Read the model definition and answer for the solid it produces. Units are mm, in the model's axes. Face numbers are marked on the shaded views. Coordinates: 2 decimals unless noted, no trailing zeros. Write each loop counter-clockwise with the first axis right and the second up, starting at its lowest first coordinate (ties: lowest second). Pieces come first, ordered by that corner, then holes.
1) Determine the mould class of the marked faces 1, 2 and 3 for opening direction Z: +Z half, -Z half, draft (parallel to the pull), parting line (faces both ways), or undercut.
2) The part is cut by section B-B (x = -10). Determine the outline of the cut face in (y, z), then the cut area to 3 significant figures.
3) Find the intervals of material crossed by line 1 (X direction, y = 6.25, z = 13.5); line 2 (X direction, y = 6, z = 13.5); line 3 (Z direction, x = -6, y = 4.75), in increasing order.
4) Each of these flat-tipped pins is pushed along its axis until it touches: pin 1 Ø2 at (x, y) = (11.5, 7) entering from +Z; pin 2 Ø1.8 at (y, z) = (5.5, 10) entering from +X; pin 3 Ø1 at (y, z) = (6, 11) entering from -X. Where does it stop, or does it pass through?
5) The part is cut by section A-A (z = 10). Determine the outline of the cut face in (x, y), then the cut area to 3 significant figures.
from build123d import *

# Parameters (mm, degrees)
F0_W      = 40
F0_H      = 20
F1_DEPTH  = 20
F2_R      = 1.75
F3_DEPTH  = 15
F4_R      = 1.75
F5_DEPTH  = 15
F6_R      = 0.5
F7_DEPTH  = 20.001
F8_R      = 2
F9_DEPTH  = 2
F12_R     = 2
F13_DEPTH = 2


with BuildPart() as f1:
    # F0 (on Top) → F1 (new body)
    with BuildSketch(Plane.XY):
        with Locations((-0.4968201369, 6.2780210599)):
            Rectangle(F0_W, F0_H)
    extrude(amount=F1_DEPTH)

    # F2 (on face) → F3 (cut)
    with BuildSketch(Plane(origin=(-20.4968201369, 0, 0), x_dir=(0, -1, 0), z_dir=(-1, 0, 0))):
        with Locations((-6.2780210599, 10)):
            Circle(F2_R)
    extrude(amount=-F3_DEPTH, mode=Mode.SUBTRACT)

    # F4 (on face) → F5 (cut)
    with BuildSketch(Plane.YZ.offset(19.5031798631)):
        with Locations((6.2780210599, 10)):
            Circle(F4_R)
    extrude(amount=-F5_DEPTH, mode=Mode.SUBTRACT)

    # F6 (on face) → F7 (cut, through all)
    with BuildSketch(Plane.XY.offset(20)):
        with Locations((-12.9968201369, 6.2780210599)):
            Circle(F6_R)
        with Locations((12.9968201369, 6.2780210599)):
            Circle(F6_R)
    extrude(amount=-F7_DEPTH, mode=Mode.SUBTRACT)

    # F8 (on face) → F9 (cut)
    with BuildSketch(Plane.XY.offset(20)):
        with Locations((-12.9968201369, 6.2780210599)):
            Circle(F8_R)
    extrude(amount=-F9_DEPTH, mode=Mode.SUBTRACT)

    # F10 (on face) → F11 (revolve, cut)
    with BuildSketch(Plane.XY.offset(18)):
        with BuildLine():
            Line((-12.9968201369, 4.2780210599), (-12.9968201369, 8.2780210599))
            ThreePointArc((-12.9968201369, 8.2780210599), (-14.9968201369, 6.2780210599), (-12.9968201369, 4.2780210599))
        make_face()
    revolve(axis=Axis((-12.9968201369, 6.2780210599, 18), (0, -1, 0)), mode=Mode.SUBTRACT)

    # F12 (on face) → F13 (cut)
    with BuildSketch(Plane.XY.offset(20)):
        with Locations((12.9968201369, 6.2780210599)):
            Circle(F12_R)
    extrude(amount=-F13_DEPTH, mode=Mode.SUBTRACT)

    # F14 (on face) → F15 (revolve, cut)
    with BuildSketch(Plane.XY.offset(18)):
        with BuildLine():
            Line((13.0087840564, 4.278056844), (13.0087840564, 8.2779852757))
            ThreePointArc((13.0087840564, 8.2779852757), (11.0088198406, 6.2780210599), (13.0087840564, 4.278056844))
        make_face()
    revolve(axis=Axis((13.0087840564, 6.2780210599, 18), (0, -1, 0)), mode=Mode.SUBTRACT)


solid = f1.part
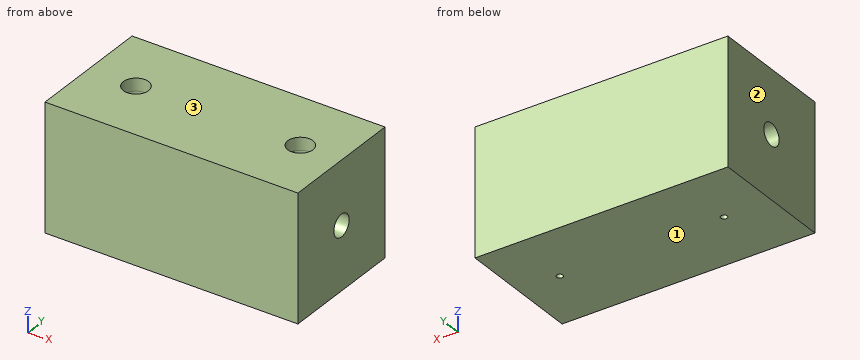
Reported:
1. face 1: -Z half
1. face 2: draft
1. face 3: +Z half
2. outline: (-3.72, 0) - (16.28, 0) - (16.28, 20) - (-3.72, 20) - close; hole circle Ø3.5 at (6.28, 10)
2. area: 390 mm2
3. line 1: x = -20.5 to -13.5, -12.5 to 12.5, 13.5 to 19.5
3. line 2: x = -20.5 to -13.41, -12.58 to 12.58, 13.41 to 19.5
3. line 3: z = 0 to 9.15, 10.85 to 20
4. pin 1: stops at z = 20
4. pin 2: stops at x = 4.5
4. pin 3: stops at x = -5.5
5. outline: (-20.5, -3.72) - (19.5, -3.72) - (19.5, 4.53) - (4.5, 4.53) - (4.5, 8.03) - (19.5, 8.03) - (19.5, 16.28) - (-20.5, 16.28) - (-20.5, 8.03) - (-5.5, 8.03) - (-5.5, 4.53) - (-20.5, 4.53) - close
5. area: 695 mm2
